```python
from build123d import *

# Parameters (mm, degrees)
SKETCH1_W           = 3.81
SKETCH1_H           = 15.24
BOSS_EXTRUDE1_DEPTH = 1.27
SKETCH2_W           = 3.81
SKETCH2_H           = 1.27
BOSS_EXTRUDE2_DEPTH = 6.35
SKETCH6_R           = 1.27
CUT_EXTRUDE1_DEPTH  = 6.35
SKETCH4_R           = 1.27
CUT_EXTRUDE2_DEPTH  = 6.35


with BuildPart() as part:
    # Sketch1 → Boss-Extrude1 (new body)
    with BuildSketch(Plane.XY):
        with Locations((1.905, 7.62)):
            Rectangle(SKETCH1_W, SKETCH1_H)
    extrude(amount=BOSS_EXTRUDE1_DEPTH)

    # Sketch2 → Boss-Extrude2 (add)
    with BuildSketch(Plane.XY.offset(1.27)):
        with Locations((1.905, 0.635)):
            Rectangle(SKETCH2_W, SKETCH2_H)
    extrude(amount=BOSS_EXTRUDE2_DEPTH)

    # Sketch6 → Cut-Extrude1 (cut)
    with BuildSketch(Plane(origin=(0, 1.27, 0), x_dir=(1, 0, 0), z_dir=(0, 1, 0))):
        with Locations(Location((1.905, -4.572, 0), (0, 0, 270))):
            Circle(SKETCH6_R)
    extrude(amount=-CUT_EXTRUDE1_DEPTH, mode=Mode.SUBTRACT)

    # Sketch4 → Cut-Extrude2 (cut)
    with BuildSketch(Plane.XY.offset(1.27)):
        with Locations((1.905, 8.466666667)):
            Circle(SKETCH4_R)
    extrude(amount=-CUT_EXTRUDE2_DEPTH, mode=Mode.SUBTRACT)


solid = part.part
```
Could you check a few things on this model? Use its own coordinates, in mm. A direction names the side the tool comes from. Round coordinates to 2 decimals unless told otherwise and drop trailing zeros. Loops run counter-clockwise (first coordinate to the right, second up) from the corner with the lowest first, then second, coordinate; pieces in that order, holes last.
Q1. On a 3-axis mill with a long thin cutter (end or side, diameter ignored), from which of +Z, -Z, +X, -X, +Y, -Y can I reach the whole of each face in a straight line? I mean faces 1 (the cylindrical face through (2.763, 0.644, 3.636)), 2 (the flat face through (2, 1.27, 3)). Say none if no direction works.
Q2. I want a section at C-C (z = 4.75). Write out the boundary of the cut face in (x, y), and give its area (3 significant figures).
Q3. For P1, Ø1, axis at x = 1, z = 2.5, coming from the +Y side, with a flat end and sliding along its axis, tell me the tip position at first contact or that it passes through.
Q4. Thinking about a two-plate mould opening in Y: for faces 3 (the flat face through (2, 10, 1.27)), 4 (the cylindrical face through (1.74, 9.726, 0.644)), 5 (the flat face through (2, 15.24, 1)), which applies, pulls with the +Y half, pulls with the -Y half, needs draft (parallel to the pull), parting line crosses it, or undercut?
Q5. Please list where these lines run through material, in increasing order: L1, parallel to Z at x = 3.55, y = 10.5; L2, parallel to Y at x = 1.75, z = 0.5.
Q6. I want a section at D-D (x = 3.5). Write out the boundary of the cut face in (y, z).
Q7. I want a section at B-B (y = 9.5). Write out the boundary of the cut face in (x, z), and give its area (3 significant figures).
Q8. I want a section at A-A (x = 2.45). Write out the boundary of the cut face in (y, z).
Answer below:
1. face 1: +Y, -Y
1. face 2: +Z, +X, -X, +Y
2. outline: (0, 0) - (0.65, 0) - (0.65, 1.27) - (0, 1.27) - close; (3.16, 0) - (3.81, 0) - (3.81, 1.27) - (3.16, 1.27) - close
2. area: 1.64 mm2
3. P1: stops at y = 1.27
4. face 3: needs draft
4. face 4: undercut
4. face 5: pulls with the +Y half
5. L1: z = 0 to 1.27
5. L2: y = 0 to 7.21, 9.73 to 15.24
6. outline: (0, 0) - (15.24, 0) - (15.24, 1.27) - (1.27, 1.27) - (1.27, 7.62) - (0, 7.62) - close
7. outline: (0, 0) - (1.17, 0) - (1.17, 1.27) - (0, 1.27) - close; (2.64, 0) - (3.81, 0) - (3.81, 1.27) - (2.64, 1.27) - close
7. area: 2.96 mm2
8. outline: (0, 0) - (7.32, 0) - (7.32, 1.27) - (1.27, 1.27) - (1.27, 3.42) - (0, 3.42) - close; (0, 5.72) - (1.27, 5.72) - (1.27, 7.62) - (0, 7.62) - close; (9.61, 0) - (15.24, 0) - (15.24, 1.27) - (9.61, 1.27) - close
